The listing builds one solid part. Answer for the finished solid, in the listing's coordinates (mm). A direction names the side the tool comes from. Round coordinates to 2 decimals unless told otherwise and drop trailing zeros. Order: outer loops, then holes, each group sorted by start corner. A loop starts at its lowest first (then second) coordinate and runs counter-clockwise, first axis right, second up. Notation, with made-up numbers: (28.25, -38) - (81.25, -38) arc R29 cw to (81.25, -17) - close; hole circle Ø4 at (67.25, 53). An arc over 180 degrees is marked (long way). One line per item, written item: value. Start each with the question number.
1. Section A-A, the plane z = 0 is taken. Give the vertices of the cut face in (x, y).
2. Section B-B, the plane x = -7.25 is taken. Give the vertices of the cut face in (y, z), then the cut area to 3 significant figures.
3. A tool of negligible diameter and unlimited length cuts with its end or side. For faces 4 (the flat face through (-9.8, 8.04, -4.13)), 5 (the flat face through (-8, 5, 2)), 6 (the flat face through (-0.1, -0.5, 0.8)), from which of +Z, -Z, +X, -X, +Y, -Y can it reach the whole face along a straight path? Write none if from no direction.
4. Flat-ended cylindrical pins translate along their axes: P1, Ø4, axis at x = 0.5, y = 3.5, coming from the +Z side; P2, Ø3.5, axis at x = 3.5, z = -5.5, coming from the -Y side; P3, Ø1.6, axis at y = 9.5, z = 2.5, coming from the -X side; P4, Ø4.5, axis at x = -0.5, z = 0, coming from the +Y side. Find the tip coordinate at first contact, or state that the pin passes through.
5. For a pull along Y with two mould halves and no side action, classify faces 1 (the cylindrical face through (-8.789, 6.311, -3.446)), 2 (the flat face through (10, 1, 0)), 3 (the flat face through (1, 2, 0)) as released by +Y, released by -Y, zero draft, split by the parting line, or undercut.
6. Section D-D, the plane z = -2.25 is taken. Give the vertices of the cut face in (x, y).
7. Section C-C, the plane y = 5.5 is taken. Give the vertices of the cut face in (x, z).
8. Straight lines are drawn through the part: line 1 (Z direction, x = -8.5, y = 5.5); line 2 (X direction, y = 12.5, z = 4); line 3 (Z direction, x = -8.45, y = 8). For each, find the intervals that lie inside material, in ascending order.
Autodesk Inventor part; units mm, degrees
ref_plane "YZ Plane" through (0, 0, 0) normal (1, 0, 0) x (0, 1, 0)
ref_plane "XZ Plane" through (0, 0, 0) normal (0, 1, 0) x (-1, 0, 0)
ref_plane "XY Plane" through (0, 0, 0) normal (0, 0, 1) x (1, 0, 0)
sketch "Sketch1" plane through (0, 0, 0) normal (0, 1, 0) x (-1, 0, 0)
  line L0 (-10, 7.5) -> (10, 7.5)
  line L1 (10, 7.5) -> (10, -7.5)
  line L2 (10, -7.5) -> (-10, -7.5)
  line L3 (-10, -7.5) -> (-10, 7.5)
  line L4 (-10, 7.5) -> (10, -7.5) construction
  line L5 (10, 7.5) -> (-10, -7.5) construction
  point P0 (0, 0)
  dimension "d0" = 20
  dimension "d1" = 15
extrude "Extrusion1" add sketch "Sketch1" along normal blind 2
sketch "Sketch2" plane through (0, 2, 0) normal (0, 1, 0) x (1, 0, 0)
  line L0 (-10, 7.5) -> (-10, -7.5)
  line L1 (-10, -7.5) -> (-8, -7.5)
  line L2 (-8, -7.5) -> (-8, 7.5)
  line L3 (-8, 7.5) -> (-10, 7.5)
  line L4 (-10, 7.5) -> (-10, -7.5)
  point P0 (0, 0)
  point P1 (-10, 0)
  point P2 (-10, 7.5)
  dimension "d4" = 2
  dimension "d5" = 15
extrude "Extrusion2" add sketch "Sketch2" along normal blind 12
sketch "Sketch3" plane through (-8, 2, 7.5) normal (1, 0, 0) x (0, 0, -1)
  circle A0 centre (7.5, 6) radius 3
  line L0 (0, 12) -> (15, 12)
  line L1 (15, 0) -> (15, 12)
  circle A1 centre (3.1699, 8.5) radius 1.2
  line L2 (0, -2) -> (0, 12)
  line L3 (0, 6) -> (15, 6) construction
  line L4 (0.8753, 9.8248) -> (14.1247, 2.1752) construction
  circle A2 centre (11.8301, 3.5) radius 1.2
  point P0 (7.5, -2)
  point P1 (7.5, 6)
  dimension "d8" = 6
  dimension "d9" = 6
  dimension "d10" = 7.5
  dimension "d11" = 2.4
  dimension "d12" = -30
  dimension "d13" = 5
  dimension "d14" = 2.4
  dimension "d15" = 5
extrude "Extrusion3" cut sketch "Sketch3" against normal blind 2
sketch "Sketch4" plane through (-10, 0, -7.5) normal (-1, 0, 0) x (0, 0, 1)
  circle A0 centre (7.5, 8) radius 3
  circle A1 centre (7.5, 8) radius 7.5
  line L0 (0, 0) -> (0, 14)
  circle A2 centre (7.5, 8) radius 12.6892
  line L1 (7.5, 8) -> (-5.1892, 8)
  line L2 (7.5, 8) -> (20.1892, 8)
  point P0 (7.5, 0)
  point P1 (15, 8)
  point P2 (0, 8)
  dimension "d18" = 15
extrude "Extrusion4" cut sketch "Sketch4" against normal blind 2 contours A1 L1 A2 L2 picked at (-3.2639, 9.6105)
sketch "Sketch5" plane through (-10, 0, -7.5) normal (-1, 0, 0) x (0, 0, 1)
  circle A0 centre (3.1699, 5.5) radius 1.2
  circle A1 centre (11.8301, 10.5) radius 1.2
  line L0 (3.1699, 5.5) -> (11.8301, 10.5) construction
  line L1 (4.2199, 3.6813) -> (12.8801, 8.6813)
  line L2 (10.7801, 12.3187) -> (2.1199, 7.3187)
  arc A2 (2.1199, 7.3187) -> (4.2199, 3.6813) centre (3.1699, 5.5) ccw
  arc A3 (12.8801, 8.6813) -> (10.7801, 12.3187) centre (11.8301, 10.5) ccw
  point P0 (7.5, 0)
  point P1 (7.5, 8)
extrude "Extrusion6" cut sketch "Sketch5" against normal blind 0.4
sketch "Sketch7" plane through (0, 0, 0) normal (0, -1, 0) x (1, 0, 0)
  line L0 (-10, -7.5) -> (-10, 7.5)
  line L1 (-10, 0.8) -> (10, 0.8)
  line L2 (10, 0.8) -> (10, -0.8)
  line L3 (10, -0.8) -> (-10, -0.8)
  line L4 (-10, -0.8) -> (-10, 0.8)
  line L5 (10, 7.5) -> (10, -7.5)
  point P0 (0, 0)
  dimension "d27" = 1.6
  dimension "d28" = 0.8
extrude "Extrusion7" add sketch "Sketch7" along normal blind 1
fillet "Fillet1" radius 2 2 edges at (10, 1, -7.5) (10, 1, 7.5)
properties part number "Trzymak"
Answer list:
1. outline: (-10, -1) - (10, -1) - (10, 2) - (-8, 2) - (-8, 5) - (-10, 5) - close; (-10, 11) - (-8, 11) - (-8, 14) - (-10, 14) - close
2. outline: (-1, -0.8) - (0, -0.8) - (0, -7.5) - (2, -7.5) - (2, 7.5) - (0, 7.5) - (0, 0.8) - (-1, 0.8) - close
2. area: 31.6 mm²
3. face 4: -X
3. face 5: +Z, -Z, +X, +Y
3. face 6: +Z, +X, -X, -Y
4. P1: stops at z = 7.5
4. P2: stops at y = 0
4. P3: stops at x = -9.6
4. P4: stops at y = 2
5. face 1: undercut
5. face 2: zero draft
5. face 3: released by +Y
6. outline: (-10, 0) - (10, 0) - (10, 2) - (-8, 2) - (-8, 6.02) - (-9.6, 6.02) - (-9.6, 4.28) - (-10, 4.28) - close; (-10, 9.98) - (-8, 9.98) - (-8, 14) - (-10, 14) - close
7. outline: (-10, -7.5) - (-8, -7.5) - (-8, -5.53) - (-9.6, -5.53) - (-9.6, -6.43) - (-10, -6.43) - close; (-10, 1.66) - (-8, 1.66) - (-8, 7.5) - (-10, 7.5) - close; (-9.6, -3.13) - (-8, -3.13) - (-8, -1.66) - (-9.6, -1.66) - close
8. line 1: z = -7.5 to -5.53, -3.13 to -1.66, 1.66 to 7.5
8. line 2: x = -9.6 to -8
8. line 3: z = -7.5 to -3, 3 to 7.5
